Geometry check sheet. Reference: the model listing, model coordinates, mm. A direction names the side the tool comes from. Give positions to 0.01 mm unless a question says otherwise; leave off trailing zeros. Loops run counter-clockwise (first coordinate to the right, second up) from the corner with the lowest first, then second, coordinate; pieces in that order, holes last. Notation, with made-up numbers: (84, 52) -> (121, 52) arc R17 ccw to (121, 61) -> close; hole circle Ø3 at (63.5, -14). An arc over 180 degrees is marked (long way). Write item = value, one per line.
```python
from build123d import *

# Parameters (mm, degrees)
SKETCH_1_R          = 35
SKETCH_1_R_2        = 10
SKETCH_1_R_3        = 1.55
SKETCH_1_R_4        = 1.7
EXTRUDE_1_DEPTH     = 12
SKETCH_2_R          = 3.25
CUT_EXTRUDE_1_DEPTH = 3.3


with BuildPart() as part:
    # 草图1 → 凸台-拉伸1 (new body)
    with BuildSketch(Plane(origin=(0, 0, 0), x_dir=(1, 0, 0), z_dir=(0, 1, 0))):
        with Locations(Location((0, 0, 0), (0, 0, 270))):
            Circle(SKETCH_1_R)
        with Locations(Location((0, 0, 0), (0, 0, 270))):
            Circle(SKETCH_1_R_2, mode=Mode.SUBTRACT)
        with Locations(Location((0, 14, 0), (0, 0, 270))):
            Circle(SKETCH_1_R_3, mode=Mode.SUBTRACT)
        with Locations(Location((12.124355653, 7, 0), (0, 0, 270))):
            Circle(SKETCH_1_R_3, mode=Mode.SUBTRACT)
        with Locations(Location((12.124355653, -7, 0), (0, 0, 270))):
            Circle(SKETCH_1_R_3, mode=Mode.SUBTRACT)
        with Locations(Location((0, -14, 0), (0, 0, 270))):
            Circle(SKETCH_1_R_3, mode=Mode.SUBTRACT)
        with Locations(Location((-12.124355653, -7, 0), (0, 0, 270))):
            Circle(SKETCH_1_R_3, mode=Mode.SUBTRACT)
        with Locations(Location((-12.124355653, 7, 0), (0, 0, 270))):
            Circle(SKETCH_1_R_3, mode=Mode.SUBTRACT)
        with Locations(Location((0, 28.5, 0), (0, 0, 270))):
            Circle(SKETCH_1_R_4, mode=Mode.SUBTRACT)
        with Locations(Location((24.681724008, 14.25, 0), (0, 0, 270))):
            Circle(SKETCH_1_R_4, mode=Mode.SUBTRACT)
        with Locations(Location((24.681724008, -14.25, 0), (0, 0, 270))):
            Circle(SKETCH_1_R_4, mode=Mode.SUBTRACT)
        with Locations(Location((0, -28.5, 0), (0, 0, 270))):
            Circle(SKETCH_1_R_4, mode=Mode.SUBTRACT)
        with Locations(Location((-24.681724008, -14.25, 0), (0, 0, 270))):
            Circle(SKETCH_1_R_4, mode=Mode.SUBTRACT)
        with Locations(Location((-24.681724008, 14.25, 0), (0, 0, 270))):
            Circle(SKETCH_1_R_4, mode=Mode.SUBTRACT)
    extrude(amount=EXTRUDE_1_DEPTH)

    # 草图2 → 切除-拉伸1 (cut)
    with BuildSketch(Plane(origin=(0, 12, 0), x_dir=(1, 0, 0), z_dir=(0, 1, 0))):
        with Locations(Location((0, 28.5, 0), (0, 0, 270))):
            Circle(SKETCH_2_R)
        with Locations(Location((24.681724008, 14.25, 0), (0, 0, 270))):
            Circle(SKETCH_2_R)
        with Locations(Location((24.681724008, -14.25, 0), (0, 0, 270))):
            Circle(SKETCH_2_R)
        with Locations(Location((0, -28.5, 0), (0, 0, 270))):
            Circle(SKETCH_2_R)
        with Locations(Location((-24.681724008, -14.25, 0), (0, 0, 270))):
            Circle(SKETCH_2_R)
        with Locations(Location((-24.681724008, 14.25, 0), (0, 0, 270))):
            Circle(SKETCH_2_R)
    extrude(amount=-CUT_EXTRUDE_1_DEPTH, mode=Mode.SUBTRACT)


solid = part.part
```
Item 1: Draft check along X on faces 1 (the cylindrical face through (27.9, 10.4, -14.7)), 2 (the cylindrical face through (-21, 6, -28)), 3 (the flat face through (-7.3, 0, 7.3)). Enter one of: +X half, -X half, draft (parallel to the pull), parting line (faces both ways), or undercut.
Answer:
face_1 = undercut
face_2 = parting line
face_3 = draft
Item 2: Section check A-A, the plane x = 0. Give the number of separate pieces and of enclosed holes in the cut face, plus the area to 3 significant figures.
Answer:
separate_pieces = 6
enclosed_holes = 0
area = 424 mm^2
Item 3: Section check D-D, the plane z = 29. Record the cut outline in (x, y).
Answer:
outline = (-19.6, 0) -> (-1.62, 0) -> (-1.62, 8.7) -> (-3.21, 8.7) -> (-3.21, 12) -> (-19.6, 12) -> close; (1.62, 0) -> (19.6, 0) -> (19.6, 12) -> (3.21, 12) -> (3.21, 8.7) -> (1.62, 8.7) -> close
Item 4: Tool access check on faces 4 (the cylindrical face through (23.17, 4.29, 15.03)), 5 (the flat face through (-1.4, 8.7, -27.1)). Record the directions out of +Z, -Z, +X, -X, +Y, -Y that give a thin tool (end or side, any length) a straight path to the whole face; none if there is none.
Answer:
face_4 = +Y, -Y
face_5 = +Y
Item 5: Gauge pin test, flat ends, axial feed: pin 1 (3 mm diameter, centred on x = 25, z = -15.5, fed in from +Y); pin 2 (3 mm diameter, centred on x = -24.68, z = -14.25, fed in from +Y); pin 3 (5 mm diameter, centred on x = 13.5, y = 9, fed in from -Z); pin 4 (4 mm diameter, centred on x = -18.5, y = 7.5, fed in from +Z). Record the tip position at first contact, or that the pin passes through.
Answer:
pin_1 = 8.7
pin_2 = through
pin_3 = -33.23
pin_4 = 30.87
Item 6: Section check B-B, the plane z = 13.5. Record the cut outline in (x, y).
Answer:
outline = (-32.29, 0) -> (-26.21, 0) -> (-26.21, 8.7) -> (-27.84, 8.7) -> (-27.84, 12) -> (-32.29, 12) -> close; (-23.16, 0) -> (-1.47, 0) -> (-1.47, 12) -> (-21.52, 12) -> (-21.52, 8.7) -> (-23.16, 8.7) -> close; (1.47, 0) -> (23.16, 0) -> (23.16, 8.7) -> (21.52, 8.7) -> (21.52, 12) -> (1.47, 12) -> close; (26.21, 0) -> (32.29, 0) -> (32.29, 12) -> (27.84, 12) -> (27.84, 8.7) -> (26.21, 8.7) -> close
Item 7: Thickness scan on L1, parallel to Z at x = 13, y = 5.25; L2, parallel to X at y = 6, z = -8; L3, parallel to X at y = 6.5, z = 0. Record the ranges inside material, lowest first. Write a range as [from, to].
Answer:
L1 = [-32.5, -8.28], [-5.72, 5.72], [8.28, 32.5]
L2 = [-34.07, -13.31], [-10.94, -6], [6, 10.94], [13.31, 34.07]
L3 = [-35, -10], [10, 35]
